```python
from build123d import *

# Parameters (mm, degrees)
SKETCH_1_W          = 20
SKETCH_1_H          = 150
EXTRUDE_1_DEPTH     = 4
CUT_EXTRUDE_1_DEPTH = 4
SKETCH_3_R          = 7
SKETCH_3_R_2        = 1.6
CUT_EXTRUDE_2_DEPTH = 76.769386958


with BuildPart() as part:
    # 草圖1 → 填料-伸長1 (new body)
    with BuildSketch(Plane.XY):
        Rectangle(SKETCH_1_W, SKETCH_1_H)
    extrude(amount=EXTRUDE_1_DEPTH)

    # 草圖2 → 除料-伸長1 (cut)
    with BuildSketch(Plane.XY.offset(4)):
        with BuildLine():
            ThreePointArc((-10, 65), (-7.071067812, 72.071067812), (0, 75))
            Line((0, 75), (-10, 75))
            Line((-10, 75), (-10, 65))
        make_face()
        with BuildLine():
            Line((10, 75), (0, 75))
            ThreePointArc((0, 75), (7.071067812, 72.071067812), (10, 65))
            Line((10, 65), (10, 75))
        make_face()
    extrude(amount=-CUT_EXTRUDE_1_DEPTH, mode=Mode.SUBTRACT)

    # 草圖3 → 除料-伸長2 (cut, through all)
    with BuildSketch(Plane.XY.offset(4)):
        with Locations((0, 63)):
            Circle(SKETCH_3_R)
        with Locations((-6, -64.632416386)):
            Circle(SKETCH_3_R_2)
        with Locations((6, -64.202233011)):
            Circle(SKETCH_3_R_2)
    extrude(amount=-CUT_EXTRUDE_2_DEPTH, mode=Mode.SUBTRACT)


solid = part.part
```
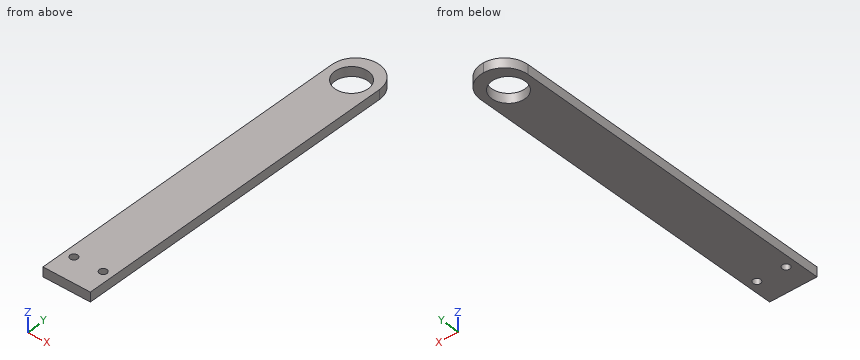
Read the model definition and answer for the solid it produces. Units are mm, in the model's axes. Coordinates: 2 decimals unless noted, no trailing zeros. Loops run counter-clockwise (first coordinate to the right, second up) from the corner with the lowest first, then second, coordinate; pieces in that order, holes last. Notation, with made-up numbers: (9.25, 36.5) -> (15.25, 36.5) arc R21 ccw to (15.25, 68.5) -> close; hole circle Ø5 at (-2.75, 27.5). An arc over 180 degrees is marked (long way). Return JSON: item names as keys, results as strings.
Item 1: Find the intervals of material crossed by probe 1 along Y at (x, z) = (6, 2.95); probe 2 along Y at (x, z) = (-3, 1.95); probe 3 along Y at (x, z) = (4.25, 1), in increasing order.
Answers:
{"probe 1": "y = -75 to -65.8, -62.6 to 59.39, 66.61 to 73", "probe 2": "y = -75 to 56.68, 69.32 to 74.54", "probe 3": "y = -75 to 57.44, 68.56 to 74.05"}
Item 2: Find section A-A (y = 63). Determine the outline of the cut face in (x, z).
Answers:
{"outline": "(-10, 0) -> (-7, 0) -> (-7, 4) -> (-10, 4) -> close; (7, 0) -> (10, 0) -> (10, 4) -> (7, 4) -> close"}
Item 3: Find section C-C (x = 2.5). Determine the outline of the cut face in (y, z), plus the area to 3 significant figures.
Answers:
{"outline": "(-75, 0) -> (56.46, 0) -> (56.46, 4) -> (-75, 4) -> close; (69.54, 0) -> (74.68, 0) -> (74.68, 4) -> (69.54, 4) -> close", "area": "546 mm2"}
Item 4: Find section D-D (z = 2.95). Determine the outline of the cut face in (x, y), plus the area to 3 significant figures.
Answers:
{"outline": "(-10, -75) -> (10, -75) -> (10, 65) arc R10 ccw to (-10, 65) -> close; hole circle Ø3.2 at (-6, -64.63); hole circle Ø14 at (0, 63); hole circle Ø3.2 at (6, -64.2)", "area": "2,790 mm2"}
Item 5: A flat-ended cylindrical pin translates along its axis: P1, Ø1.5, axis at x = -1.5, z = 2.5, coming from the +Y side. Find the tip coordinate at first contact, or state that the pin passes through.
Answers:
{"P1": "stops at y = 74.97"}
Item 6: Find section B-B (x = -5.75). Determine the outline of the cut face in (y, z).
Answers:
{"outline": "(-75, 0) -> (-66.21, 0) -> (-66.21, 4) -> (-75, 4) -> close; (-63.05, 0) -> (59.01, 0) -> (59.01, 4) -> (-63.05, 4) -> close; (66.99, 0) -> (73.18, 0) -> (73.18, 4) -> (66.99, 4) -> close"}
